from build123d import *

# Parameters (mm, degrees)
ESBO_O1_R                  = 50
RESSALTO_EXTRUS_O1_DEPTH   = 2
ESBO_O2_R                  = 2.75
CORTE_EXTRUS_O1_DEPTH      = 2
CORTE_EXTRUS_O2_DEPTH      = 1
CORTE_EXTRUS_O2_DEPTH_BACK = 10
ESBO_O5_R                  = 1.5
ESBO_O5_R_2                = 1.75
CORTE_EXTRUS_O3_DEPTH      = 10


with BuildPart() as part:
    # Esboço1 → Ressalto-extrusão1 (new body)
    with BuildSketch(Plane.XY):
        Circle(ESBO_O1_R)
    extrude(amount=RESSALTO_EXTRUS_O1_DEPTH)

    # Esboço2 → Corte-extrusão1 (cut)
    with BuildSketch(Plane.XY.offset(2)):
        with Locations((-29, -34.409301068)):
            Circle(ESBO_O2_R)
        with Locations((29, -34.409301068)):
            Circle(ESBO_O2_R)
        with Locations((-38.824197531, 22.752619324)):
            Circle(ESBO_O2_R)
        with Locations((38.824197531, 22.752619324)):
            Circle(ESBO_O2_R)
    extrude(amount=-CORTE_EXTRUS_O1_DEPTH, mode=Mode.SUBTRACT)

    # Esboço4 → Corte-extrusão2 (cut, two sides)
    with BuildSketch(Plane.XY.offset(2)) as corte_extrus_o2_sk:
        Polygon((-40.723859979, -38.409301068), (44.57073926, -38.409301068), (1.923439641, -68.002213614), align=None)
    extrude(amount=CORTE_EXTRUS_O2_DEPTH, mode=Mode.SUBTRACT)
    extrude(corte_extrus_o2_sk.sketch, amount=-CORTE_EXTRUS_O2_DEPTH_BACK, mode=Mode.SUBTRACT)

    # Esboço5 → Corte-extrusão3 (cut)
    with BuildSketch(Plane(origin=(0, 0, 0), x_dir=(-1, 0, 0), z_dir=(0, 0, -1))):
        with Locations((-27.91, -18.86)):
            Circle(ESBO_O5_R)
        with Locations((27.7, -18.86)):
            Circle(ESBO_O5_R)
        with Locations((27.7, 0.44)):
            Circle(ESBO_O5_R)
        with Locations((-27.91, 0.44)):
            Circle(ESBO_O5_R)
        with Locations((25.5, 31.36)):
            Circle(ESBO_O5_R_2)
        with Locations((-0.05, 27.79)):
            Circle(ESBO_O5_R_2)
        with Locations((-25.5, 31.36)):
            Circle(ESBO_O5_R_2)
    extrude(amount=-CORTE_EXTRUS_O3_DEPTH, mode=Mode.SUBTRACT)


solid = part.part
The model under review builds one solid part; all positions refer to its coordinate system, in mm. Coordinates: 2 decimals unless noted, no trailing zeros. Loops run counter-clockwise (first coordinate to the right, second up) from the corner with the lowest first, then second, coordinate; pieces in that order, holes last. Notation, with made-up numbers: M 79.25,54 L 83.25,54 A29 cw 83.25,75 Z; hole C 35,-34.75 d5. An arc over 180 degrees is marked long. Put each result on its own line as item: value. Start each with the question number.
Q1. The part is to be moulded in two halves that separate along X. For faces 1 (the cylindrical face through (1.71, 49.97, 0.99)), 2 (the flat face through (-1, 6, 2)), 3 (the cylindrical face through (-29.13, 0.89, 0.99)), say which applies: +X half, -X half, draft (parallel to the pull), parting line (faces both ways), or undercut.
Q2. Add section B-B (x = -40.5). Write out the cut boundary in (y, z), and give its area (3 significant figures).
Q3. Add section A-A (y = -18.86). Write out the cut boundary in (x, z), and give its area (3 significant figures).
Q4. Clearance check with flat-ended pins moving along their axes: pin 1 (3 mm diameter, centred on x = -25.5, y = 31.36, fed in from +Z); pin 2 (1 mm diameter, centred on y = -12.5, z = 1, fed in from +X). State where each tip first meets the part, or that it passes through.
Q5. Add section D-D (y = 27.79). Write out the cut boundary in (x, z), and give its area (3 significant figures).
Q6. Wall thickness on line 1 (Y direction, x = 0.05, z = 0.75); line 2 (Y direction, x = 29, z = 1.85); line 3 (Y direction, x = 27.91, z = 1.4): over which ranges is each line inside the solid? List them lowest first.
Q7. Add section C-C (z = 0.5). Count the separate pieces of the cut face and the enclosed holes in it, and give its area (3 significant figures).
Answers:
1. face 1: parting line
1. face 2: draft
1. face 3: undercut
2. outline: M -29.32,0 L 20.57,0 L 20.57,2 L -29.32,2 Z; M 24.93,0 L 29.32,0 L 29.32,2 L 24.93,2 Z
2. area: 109 mm^2
3. outline: M -46.31,0 L -29.2,0 L -29.2,2 L -46.31,2 Z; M -26.2,0 L 26.41,0 L 26.41,2 L -26.2,2 Z; M 29.41,0 L 46.31,0 L 46.31,2 L 29.41,2 Z
3. area: 173 mm^2
4. pin 1: passes through
4. pin 2: stops at x = 48.54
5. outline: M -41.57,0 L -1.7,0 L -1.7,2 L -41.57,2 Z; M 1.8,0 L 41.57,0 L 41.57,2 L 1.8,2 Z
5. area: 159 mm^2
6. line 1: y = -38.41 to 26.04, 29.54 to 50
6. line 2: y = -38.41 to -37.16, -31.66 to -19.89, -17.83 to -0.59, 1.47 to 40.73
6. line 3: y = -38.41 to -36.93, -31.88 to -20.36, -17.36 to -1.06, 1.94 to 41.49
7. separate pieces: 1
7. enclosed holes: 11
7. area: 7,190 mm^2
